```python
from build123d import *

# Parameters (mm, degrees)
F0_R     = 7
F1_DEPTH = 2
F2_R     = 5.75
F3_DEPTH = 21
F4_R     = 3
F5_DEPTH = 20
F6_R     = 6.6303140267
F6_R_2   = 4.5
F7_DEPTH = 1.9
F8_W     = 5
F8_H     = 8
F9_DEPTH = 0.3


with BuildPart() as f1:
    # F0 (on Front) → F1 (new body)
    with BuildSketch(Plane.XZ):
        Circle(F0_R)
    extrude(amount=-F1_DEPTH)

    # F2 (on face) → F3 (join)
    with BuildSketch(Plane(origin=(0, 2, 0), x_dir=(-1, 0, 0), z_dir=(0, 1, 0))):
        Circle(F2_R)
    extrude(amount=F3_DEPTH)

    # F4 (on face) → F5 (cut)
    with BuildSketch(Plane.XZ):
        Circle(F4_R)
    extrude(amount=-F5_DEPTH, mode=Mode.SUBTRACT)

    # F6 (on face) → F7 (cut)
    with BuildSketch(Plane.XZ):
        Circle(F6_R)
        Circle(F6_R_2, mode=Mode.SUBTRACT)
    extrude(amount=-F7_DEPTH, mode=Mode.SUBTRACT)

    # F8 (on Top) → F9 (join, symmetric)
    with BuildSketch(Plane.XY):
        with Locations((0, 26)):
            Rectangle(F8_W, F8_H)
    extrude(amount=F9_DEPTH, both=True)


solid = f1.part
```
For this review, take the finished solid that the model builds, in its own axes (mm). A direction names the side the tool comes from. Coordinates: 2 decimals unless noted, no trailing zeros. Order: outer loops, then holes, each group sorted by start corner. A loop starts at its lowest first (then second) coordinate and runs counter-clockwise, first axis right, second up. Notation, with made-up numbers: (33.25, -2) -> (82.25, -2) arc R26 cw to (82.25, 26) -> close; hole circle Ø11 at (-14.75, 32). An arc over 180 degrees is marked (long way). Answer as CSV lines item,"result".
Q1. For faces 5 (the face through (-6.624, 0.937, 0.292)), 6 (the face through (0, 27, -0.3)), 7 (the face through (0.75, 12.35, 5.7)), list the 3-axis set-ups (+Z, -Z, +X, -X, +Y, -Y) from which the entire face can be reached by the end or side of a thin tool; tool diameter is ignored.
Model answer:
face 5,"-Y"
face 6,"-Z, +X, -X, +Y"
face 7,"+Y"
Q2. We need section B-B (x = 0). State the section outline as (y, z) points, plus the area to 3 significant figures.
Model answer:
outline,"(0, -7) -> (2, -7) -> (2, -5.75) -> (23, -5.75) -> (23, -0.3) -> (30, -0.3) -> (30, 0.3) -> (23, 0.3) -> (23, 5.75) -> (2, 5.75) -> (2, 7) -> (0, 7) -> (0, 6.63) -> (1.9, 6.63) -> (1.9, 4.5) -> (0, 4.5) -> (0, 3) -> (20, 3) -> (20, -3) -> (0, -3) -> (0, -4.5) -> (1.9, -4.5) -> (1.9, -6.63) -> (0, -6.63) -> close"
area,"146 mm2"
Q3. We need section C-C (y = 8.5). State the section outline as (x, z) points, plus the area to 3 significant figures.
Model answer:
outline,"circle Ø11.5 at (0, 0); hole circle Ø6 at (0, 0)"
area,"75.6 mm2"
Q4. Wall thickness on line 1 along Z through (x, y) = (0, 0.6); line 2 along Z through (x, y) = (0, 6); line 3 along Y through (x, z) = (0.75, -1): over which ranges is each line inside the solid? List them lowest first. Write a range as [from, to].
Model answer:
line 1,"z = [-7, -6.63], [-4.5, -3], [3, 4.5], [6.63, 7]"
line 2,"z = [-5.75, -3], [3, 5.75]"
line 3,"y = [20, 23]"
Q5. We need section A-A (z = 0). State the section outline as (x, y) points.
Model answer:
outline,"(-7, 0) -> (-6.63, 0) -> (-6.63, 1.9) -> (-4.5, 1.9) -> (-4.5, 0) -> (-3, 0) -> (-3, 20) -> (3, 20) -> (3, 0) -> (4.5, 0) -> (4.5, 1.9) -> (6.63, 1.9) -> (6.63, 0) -> (7, 0) -> (7, 2) -> (5.75, 2) -> (5.75, 23) -> (2.5, 23) -> (2.5, 30) -> (-2.5, 30) -> (-2.5, 23) -> (-5.75, 23) -> (-5.75, 2) -> (-7, 2) -> close"
Q6. We need section D-D (y = 25.5). State the section outline as (x, z) points.
Model answer:
outline,"(-2.5, -0.3) -> (2.5, -0.3) -> (2.5, 0.3) -> (-2.5, 0.3) -> close"
Q7. Draft analysis for pull direction Z (two halves, no side actions). For faces 1 (the face through (6.466, 0.986, -2.681)), 2 (the face through (1, 0, -3)), 3 (the face through (0, 27, 0.3)), 4 (the face through (-3, 10, 0)), state which applies: released by +Z, released by -Z, zero draft, split by the parting line, or undercut.
Model answer:
face 1,"split by the parting line"
face 2,"zero draft"
face 3,"released by +Z"
face 4,"undercut"
Q8. Clearance check with flat-ended pins moving along their axes: pin 1 Ø4 at (x, y) = (1, 28) entering from +Z; pin 2 Ø1.5 at (x, y) = (-1.5, 10.5) entering from -Z; pin 3 Ø6 at (x, y) = (-3, 7.5) entering from +Z. State where each tip first meets the part, or that it passes through.
Model answer:
pin 1,"stops at z = 0.3"
pin 2,"stops at z = -5.7"
pin 3,"stops at z = 5.75"
